Part model, mm, in its own coordinate system. A direction names the side the tool comes from. Round coordinates to 2 decimals unless told otherwise and drop trailing zeros. Order: outer loops, then holes, each group sorted by start corner. A loop starts at its lowest first (then second) coordinate and runs counter-clockwise, first axis right, second up. Notation, with made-up numbers: M -38.75,49.25 L -19.75,49.25 A26 cw -19.75,83.25 Z; hole C -7.75,39.25 d3. An arc over 180 degrees is marked long. One line per question, with ' | ' between items.
from build123d import *

# Parameters (mm, degrees)
SKETCH1_R                = 15
BOSS_EXTRUDE1_DEPTH      = 14
SKETCH4_R                = 14
CUT_EXTRUDE1_DEPTH       = 15
SKETCH3_R                = 15
SKETCH3_R_2              = 12
BOSS_EXTRUDE2_DEPTH      = 3
SKETCH6_R                = 3.25
SKETCH6_R_2              = 1.75
BOSS_EXTRUDE4_DEPTH      = 17
FILLET1_R                = 5
CIRPATTERN2_COUNT        = 3
FILLET1_OF_CIRPATTERN2_R = 5


with BuildPart() as part:
    # Sketch1 → Boss-Extrude1 (new body)
    with BuildSketch(Plane.XY):
        Circle(SKETCH1_R)
    extrude(amount=BOSS_EXTRUDE1_DEPTH)

    # Sketch4 → Cut-Extrude1 (cut, through all)
    with BuildSketch(Plane(origin=(0, 0, 0), x_dir=(-1, 0, 0), z_dir=(0, 0, -1))):
        Circle(SKETCH4_R)
    extrude(amount=-CUT_EXTRUDE1_DEPTH, mode=Mode.SUBTRACT)

    # Sketch3 → Boss-Extrude2 (add)
    with BuildSketch(Plane(origin=(0, 0, 0), x_dir=(-1, 0, 0), z_dir=(0, 0, -1))):
        Circle(SKETCH3_R)
        Circle(SKETCH3_R_2, mode=Mode.SUBTRACT)
    extrude(amount=BOSS_EXTRUDE2_DEPTH)

    # Sketch6 → Boss-Extrude4 (add)
    with BuildSketch(Plane.XY.offset(14)):
        with Locations((0, 17.25)):
            Circle(SKETCH6_R)
        with Locations((0, 17.25)):
            Circle(SKETCH6_R_2, mode=Mode.SUBTRACT)
    boss_extrude4 = extrude(amount=-BOSS_EXTRUDE4_DEPTH)

    # Fillet1
    fillet1_edges = [part.edges().sort_by_distance(p)[0] for p in [
        (2.181099234, 14.84057971, 7),
        (-2.181099234, 14.84057971, 7),
    ]]
    fillet(fillet1_edges, radius=FILLET1_R)

    # CirPattern2: Boss-Extrude4 ×3 about axis
    cirpattern2_axis = Axis((0, 0, 0), (0, 0, 1))
    for i in range(1, CIRPATTERN2_COUNT):
        add(boss_extrude4.rotate(cirpattern2_axis, i * 360 / CIRPATTERN2_COUNT))

    # Fillet1 of CirPattern2
    fillet1_of_cirpattern2_edges = [part.edges().sort_by_distance(p)[0] for p in [
        (-13.942868653, -5.531402511, 7),
        (-11.761769419, -9.3091772, 7),
        (11.761769419, -9.3091772, 7),
        (13.942868653, -5.531402511, 7),
    ]]
    fillet(fillet1_of_cirpattern2_edges, radius=FILLET1_OF_CIRPATTERN2_R)


solid = part.part
1) Saw through at A-A (x = 0). List the corners of the cut face in (y, z).
The answers:
outline: M -15,-3 L -12,-3 L -12,0 L -14,0 L -14,14 L -15,14 Z; M 12,-3 L 15.5,-3 L 15.5,14 L 14,14 L 14,0 L 12,0 Z; M 19,-3 L 20.5,-3 L 20.5,14 L 19,14 Z
2) Saw through at B-B (y = 0). List the corners of the cut face in (x, z).
The answers:
outline: M -15,-3 L -12,-3 L -12,0 L -14,0 L -14,14 L -15,14 Z; M 12,-3 L 15,-3 L 15,14 L 14,14 L 14,0 L 12,0 Z
3) Which spindle directions (+Z, -Z, +X, -X, +Y, -Y) get a long thin tool onto all of the face, cutting with end or side? Do faces 4 (the face through (-12.932, -5.362, 6.902)), 5 (the face through (4, 14, 14)). Say none if no direction does.
The answers:
face 4: +Z | face 5: +Z, +X, -X, +Y, -Y
4) Probe line 1 (Y direction, x = 0, z = 1.25); line 2 (Y direction, x = 0, z = -2); line 3 (X direction, y = -8, z = 5.5). List the from-to ranges inside material, lowest first. Write a range as [from, to].
The answers:
line 1: y = [-15, -14], [14, 15.5], [19, 20.5] | line 2: y = [-15, -12], [12, 15.5], [19, 20.5] | line 3: x = [-18.13, -16.57], [-13.3, -11.49], [11.49, 13.3], [16.57, 18.13]
5) Saw through at C-C (y = -9.5). List the corners of the cut face in (x, z).
The answers:
outline: M -18.07,-3 L -16.45,-3 L -16.45,14 L -18.07,14 Z; M -13.42,-3 L -7.33,-3 L -7.33,0 L -10.28,0 L -10.28,14 L -13.42,14 Z; M 7.33,-3 L 13.42,-3 L 13.42,14 L 10.28,14 L 10.28,0 L 7.33,0 Z; M 16.45,-3 L 18.07,-3 L 18.07,14 L 16.45,14 Z
6) Drop flat-ended pins along their axis: pin 1 (4 mm diameter, centred on y = -3, z = 11.5, fed in from +X); pin 2 (8 mm diameter, centred on x = -7, z = 6.5, fed in from +Y); pin 3 (2 mm diameter, centred on y = -11, z = 6, fed in from +X); pin 4 (6 mm diameter, centred on y = -9, z = 1, fed in from +X). Give the stop position or say it passes through.
The answers:
pin 1: stops at x = 15.87 | pin 2: stops at y = 18.5 | pin 3: stops at x = 17.88 | pin 4: stops at x = 18.19
7) Saw through at D-D (x = -7.5). List the corners of the cut face in (y, z), plus the area to 3 significant figures.
The answers:
outline: M -12.99,-3 L -9.37,-3 L -9.37,0 L -11.82,0 L -11.82,14 L -12.99,14 Z; M 9.37,-3 L 12.99,-3 L 12.99,14 L 11.82,14 L 11.82,0 L 9.37,0 Z | area: 54.5 mm²
8) Two-plate mould, pull along Y, no slides. Class faces 1 (the face through (-16.687, -8.548, 5.619)), 2 (the face through (17.72, -10.31, 5.62)), 3 (the face through (-12, -2, -3)): released by +Y, released by -Y, zero draft, split by the parting line, or undercut.
The answers:
face 1: undercut | face 2: split by the parting line | face 3: zero draft
